```python
from build123d import *

# Parameters (mm, degrees)
BOX018_W     = 6
BOX018_H     = 3.5
BOX018_DEPTH = 3
BOX010_W     = 8
BOX010_H     = 5.5
BOX010_DEPTH = 1
BOX011_W     = 3
BOX011_H     = 1.5
BOX011_DEPTH = 2
BOX009_W     = 6
BOX009_H     = 3.5
BOX009_DEPTH = 2
BOX004_W     = 40
BOX004_H     = 30
BOX004_DEPTH = 2


with BuildPart() as cube016:
    # Box018 → Box018 (new body)
    with BuildSketch(Plane(origin=(22, 12, 11), x_dir=(1, 0, 0), z_dir=(0, 0, 1))):
        with Locations((3, 1.75)):
            Rectangle(BOX018_W, BOX018_H)
    extrude(amount=BOX018_DEPTH)


with BuildPart() as cube008:
    # Box010 → Box010 (new body)
    with BuildSketch(Plane(origin=(10, 11, 10), x_dir=(1, 0, 0), z_dir=(0, 0, 1))):
        with Locations((4, 2.75)):
            Rectangle(BOX010_W, BOX010_H)
    extrude(amount=BOX010_DEPTH)


with BuildPart() as cube009:
    # Box011 → Box011 (new body)
    with BuildSketch(Plane(origin=(12.5, 13, 12), x_dir=(1, 0, 0), z_dir=(0, 0, 1))):
        with Locations((1.5, 0.75)):
            Rectangle(BOX011_W, BOX011_H)
    extrude(amount=BOX011_DEPTH)


with BuildPart() as fusion002:
    # Box009 → Box009 (new body)
    with BuildSketch(Plane(origin=(11, 12, 10), x_dir=(1, 0, 0), z_dir=(0, 0, 1))):
        with Locations((3, 1.75)):
            Rectangle(BOX009_W, BOX009_H)
    extrude(amount=BOX009_DEPTH)

    # Fusion002: union Cube008, Cube009
    add(cube008.part)
    add(cube009.part)


with BuildPart() as top:
    # Box004 → Box004 (new body)
    with BuildSketch(Plane.XY.offset(11)):
        with Locations((20, 15)):
            Rectangle(BOX004_W, BOX004_H)
    extrude(amount=BOX004_DEPTH)

    # Cut002: cut Fusion002
    add(fusion002.part, mode=Mode.SUBTRACT)

    # Cut005: cut Cube016
    add(cube016.part, mode=Mode.SUBTRACT)


solid = top.part
```
Design review of the part built by this model. Coordinates are the model's own, in mm. A direction names the side the tool comes from. Round coordinates to 2 decimals unless told otherwise and drop trailing zeros. Write each loop counter-clockwise with the first axis right and the second up, starting at its lowest first coordinate (ties: lowest second). Pieces come first, ordered by that corner, then holes.
Item 1: We need section B-B on y = 15. Write out the cut boundary in (x, z), and give its area (3 significant figures).
Item 2: Clearance check with a flat-ended pin moving along its axis: pin 1 Ø1 at (x, y) = (14, 13) entering from -Z. State where the tip first meets the part, or that it passes through.
Item 3: The part is to be moulded in two halves that separate along X. For faces 1 (the flat face through (20, 15, 13)), 2 (the flat face through (28, 14, 12)), 3 (the flat face through (40, 15, 12)), say which applies: +X half, -X half, draft (parallel to the pull), parting line (faces both ways), or undercut.
Item 4: For probe 1 along Y at (x, z) = (15, 12.1); probe 2 along Y at (x, z) = (22.5, 11.6); probe 3 along Z at (x, y) = (13.5, 12.5), list the stretches that pass through material, from the lowest coordinate up.
Item 5: We need section C-C on x = 12. Write out the cut boundary in (y, z), and give its area (3 significant figures).
Item 6: We need section A-A on z = 12.55. Write out the cut boundary in (x, y).
Item 7: For faces 4 (the flat face through (20, 0, 12)), 5 (the flat face through (25, 15.5, 12)), 6 (the flat face through (14, 15.5, 11.5)), list the 3-axis set-ups (+Z, -Z, +X, -X, +Y, -Y) from which the entire face can be reached by the end or side of a thin tool; tool diameter is ignored.
Returned:
1. outline: (0, 11) - (11, 11) - (11, 12) - (17, 12) - (17, 11) - (22, 11) - (22, 13) - (0, 13) - close; (28, 11) - (40, 11) - (40, 13) - (28, 13) - close
1. area: 62.0 mm2
2. pin 1: stops at z = 12
3. face 1: draft
3. face 2: undercut
3. face 3: +X half
4. probe 1: y = 0 to 13, 14.5 to 30
4. probe 2: y = 0 to 12, 15.5 to 30
4. probe 3: z = 12 to 13
5. outline: (0, 11) - (12, 11) - (12, 12) - (15.5, 12) - (15.5, 11) - (30, 11) - (30, 13) - (0, 13) - close
5. area: 56.5 mm2
6. outline: (0, 0) - (40, 0) - (40, 30) - (0, 30) - close; hole (12.5, 13) - (15.5, 13) - (15.5, 14.5) - (12.5, 14.5) - close; hole (22, 12) - (28, 12) - (28, 15.5) - (22, 15.5) - close
7. face 4: +Z, -Z, +X, -X, -Y
7. face 5: +Z, -Z
7. face 6: -Z
